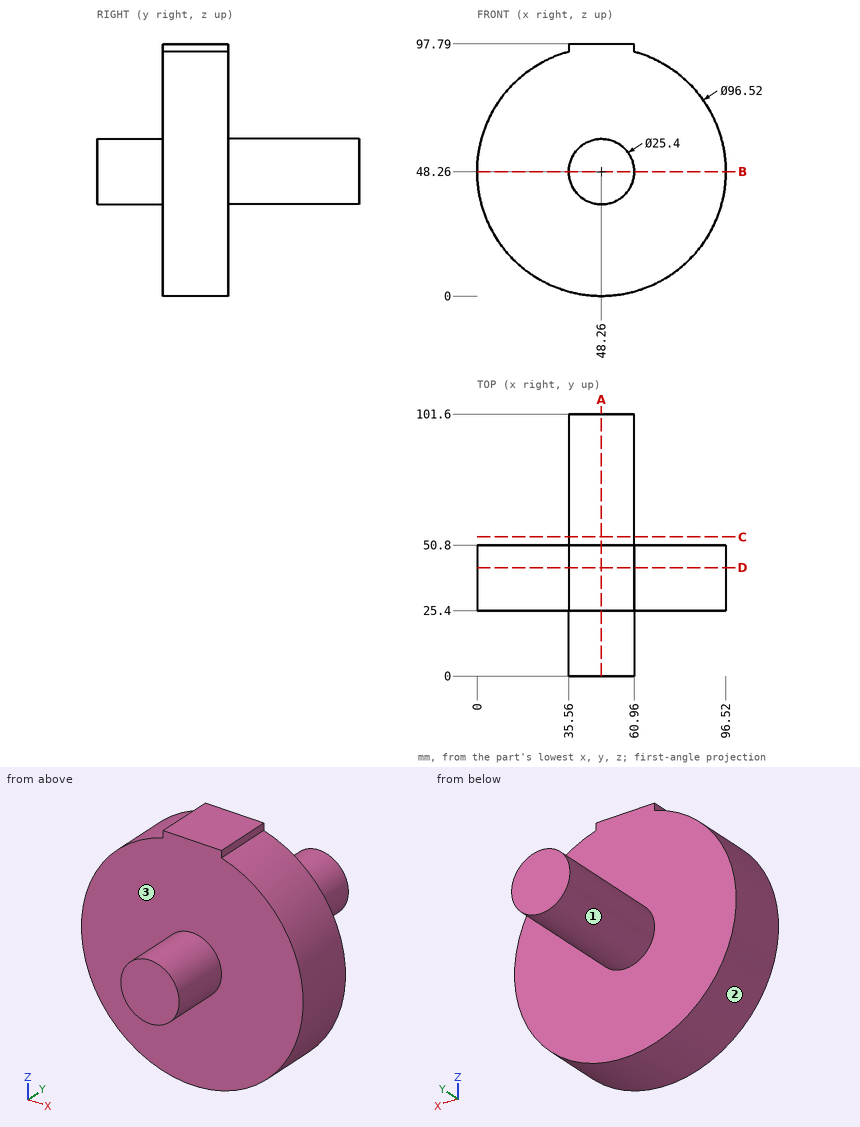
Here's the drawing with two shaded views (mm, measured from the low corner). I have some questions. A direction names the side the tool comes from. Coordinates: 2 decimals unless noted, no trailing zeros. Loops run counter-clockwise (first coordinate to the right, second up) from the corner with the lowest first, then second, coordinate; pieces in that order, holes last. Notation, with made-up numbers: M 57.25,-30 L 116.25,-30 A27 cw 116.25,-3 Z; hole C -21,61 d6. An arc over 180 degrees is marked long. Put each result on its own line as item: value. Start each with the question number.
(1) Which directions (+Z, -Z, +X, -X, +Y, -Y) give clear straight access to the entire face, cutting with the end or side of a thin tool? Please do the marked faces 1, 2 and 3.
(2) Imagine slicing it at C-C on y = 54. List the corners of the cut face in (x, z) for me.
(3) Will these pins go through, and if not, where does the flat tip stop? pin 1 Ø10 at (x, z) = (12.5, 73.5) entering from -Y; pin 2 Ø1.5 at (y, z) = (42, 96.5) entering from +X; pin 3 Ø2 at (x, y) = (50, 90) entering from +Z.
(4) Imagine slicing it at D-D on y = 42. List the corners of the cut face in (x, z) for me.
(5) Imagine slicing it at B-B on z = 48.26. List the corners of the cut face in (x, y) for me.
(6) Imagine slicing it at A-A on x = 48.26. List the corners of the cut face in (y, z) for me.
(7) I need wall thicknesses on probe 1 along Y at (x, z) = (25.5, 76); probe 2 along X at (y, z) = (54.5, 55.5); probe 3 along Z at (x, y) = (65, 37). Which ranges of each line are inside material? Lowest first, please.
Worked answers:
1. face 1: +Y
1. face 2: +Y, -Y
1. face 3: -Y
2. outline: C 48.26,48.26 d25.4
3. pin 1: stops at y = 25.4
3. pin 2: stops at x = 60.96
3. pin 3: stops at z = 60.94
4. outline: M 35.56,94.82 A48.26 ccw long 60.96,94.82 L 60.96,97.79 L 35.56,97.79 Z
5. outline: M 0,25.4 L 35.56,25.4 L 35.56,0 L 60.96,0 L 60.96,25.4 L 96.52,25.4 L 96.52,50.8 L 60.96,50.8 L 60.96,101.6 L 35.56,101.6 L 35.56,50.8 L 0,50.8 Z
6. outline: M 0,35.56 L 25.4,35.56 L 25.4,0 L 50.8,0 L 50.8,35.56 L 101.6,35.56 L 101.6,60.96 L 50.8,60.96 L 50.8,97.79 L 25.4,97.79 L 25.4,60.96 L 0,60.96 Z
7. probe 1: y = 25.4 to 50.8
7. probe 2: x = 37.83 to 58.69
7. probe 3: z = 3 to 93.52
